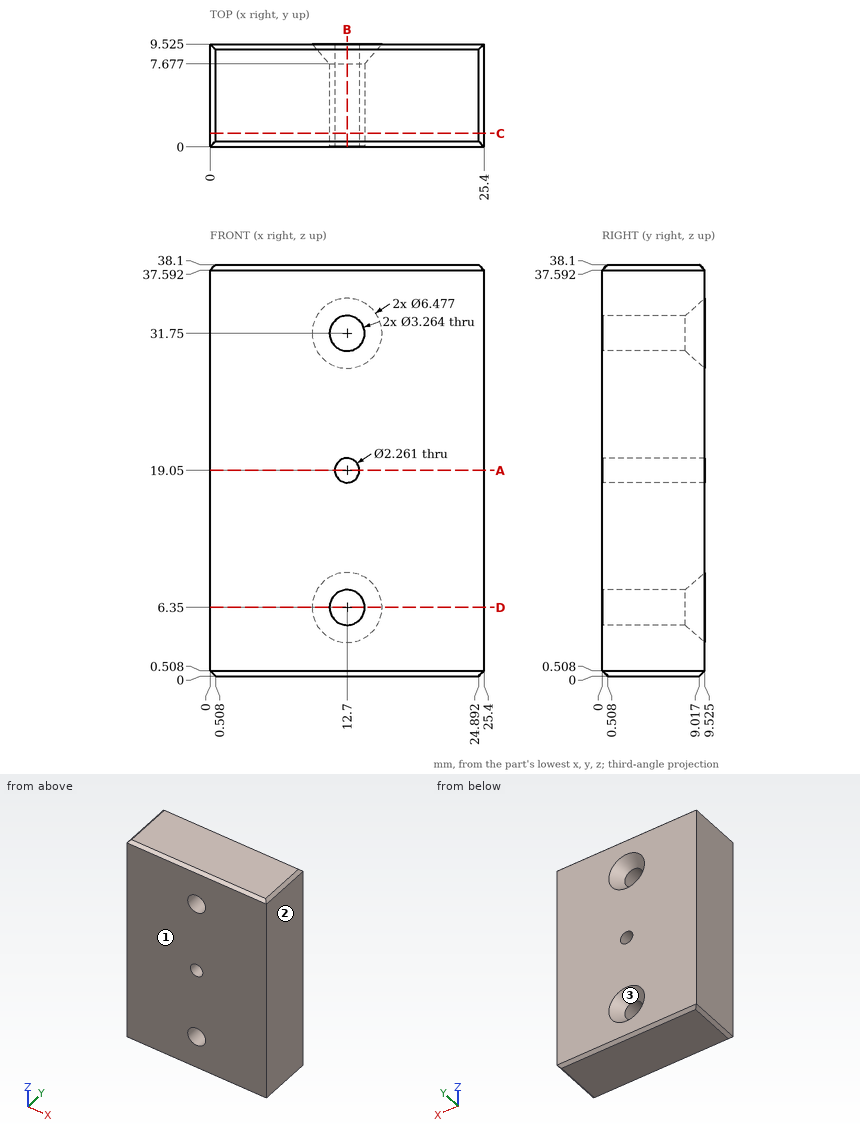
Print and shaded views of the part. All mm, measured from the part's lowest x, y and z. Round coordinates to 2 decimals unless told otherwise and drop trailing zeros. Order: outer loops, then holes, each group sorted by start corner. A loop starts at its lowest first (then second) coordinate and runs counter-clockwise, first axis right, second up.
Q1. Slice it at D-D (z = 6.35). Write the cut outline in (x, y) (1 decimal).
Q2. Slice it at A-A (z = 19.05). Write the cut outline in (x, y) (1 decimal), and give its area (3 significant figures).
Q3. Slice it at C-C (y = 1.25). Write the cut outline in (x, z).
Q4. Slice it at B-B (x = 12.7). Write the cut outline in (y, z) (1 decimal).
Q5. Drop a flat-ended pin along its axis: pin 1 (4 mm diameter, centred on x = 12.7, z = 31.75, fed in from +Y). Give the stop position or say it passes through.
Q6. Wall check: L1, parallel to Z at x = 12.7, y = 4; L2, parallel to X at y = 5.5, z = 19.05; L3, parallel to X at y = 2.75, z = 31.75. Give the ranges that are in metal, low to high.
Q7. Two-plate mould, pull along X, no slides. Class the marked faces 1, 2 and 3: pulls with the +X half, pulls with the -X half, needs draft (parallel to the pull), parting line crosses it, or undercut.
Results below:
1. outline: (0, 0) - (11.1, 0) - (11.1, 7.7) - (9.5, 9.5) - (0, 9.5) - close; (14.3, 0) - (25.4, 0) - (25.4, 9.5) - (15.9, 9.5) - (14.3, 7.7) - close
2. outline: (0, 0) - (11.6, 0) - (11.6, 9.5) - (0, 9.5) - close; (13.8, 0) - (25.4, 0) - (25.4, 9.5) - (13.8, 9.5) - close
2. area: 220 mm2
3. outline: (0, 0.51) - (0.51, 0) - (24.89, 0) - (25.4, 0.51) - (25.4, 37.59) - (24.89, 38.1) - (0.51, 38.1) - (0, 37.59) - close; hole circle Ø3.26 at (12.7, 6.35); hole circle Ø3.26 at (12.7, 31.75); hole circle Ø2.26 at (12.7, 19.05)
4. outline: (0, 0.5) - (0.5, 0) - (9, 0) - (9.5, 0.5) - (9.5, 3.1) - (7.7, 4.7) - (0, 4.7) - close; (0, 8) - (7.7, 8) - (9.5, 9.6) - (9.5, 17.9) - (0, 17.9) - close; (0, 20.2) - (9.5, 20.2) - (9.5, 28.5) - (7.7, 30.1) - (0, 30.1) - close; (0, 33.4) - (7.7, 33.4) - (9.5, 35) - (9.5, 37.6) - (9, 38.1) - (0.5, 38.1) - (0, 37.6) - close
5. pin 1: stops at y = 8.1
6. L1: z = 0 to 4.72, 7.98 to 17.92, 20.18 to 30.12, 33.38 to 38.1
6. L2: x = 0 to 11.57, 13.83 to 25.4
6. L3: x = 0 to 11.07, 14.33 to 25.4
7. face 1: needs draft
7. face 2: pulls with the +X half
7. face 3: undercut
